```python
from build123d import *

# Parameters (mm, degrees)
PAD_DEPTH       = 3
SKETCH001_W     = 2
SKETCH001_H     = 6
POCKET_DEPTH    = 5
PAD001_DEPTH    = 2.2
SKETCH003_R     = 1.571244
POCKET001_DEPTH = 5


with BuildPart() as part:
    # Sketch → Pad (new body)
    with BuildSketch(Plane.XY):
        Polygon((0, -50), (9.32, -50), (9.32, 40), (35, 55), (35, 120), (0, 120), align=None)
    extrude(amount=PAD_DEPTH)

    # Sketch001 (on Face7 of Pad) → Pocket (cut)
    with BuildSketch(Plane(origin=(0, 0, 0), x_dir=(1, 0, 0), z_dir=(0, 0, -1))):
        with Locations((1, 0)):
            Rectangle(SKETCH001_W, SKETCH001_H)
    pocket = extrude(amount=-POCKET_DEPTH, mode=Mode.SUBTRACT)

    # Sketch002 (on Face3 of Pocket) → Pad001 (join)
    with BuildSketch(Plane.YZ.offset(9.32)):
        Polygon((-3, 0), (-3, 40), (-12, 40), (-34, 0), align=None)
    pad001 = extrude(amount=PAD001_DEPTH)

    # Sketch003 (on Face18 of Pad001) → Pocket001 (cut)
    with BuildSketch(Plane.YZ.offset(11.52)):
        with Locations((-8.751605, 34.485332)):
            Circle(SKETCH003_R)
    pocket001 = extrude(amount=-POCKET001_DEPTH, mode=Mode.SUBTRACT)

    # Mirrored: Pocket, Pad001, Pocket001 across XZ
    add(pocket.mirror(Plane.XZ), mode=Mode.SUBTRACT)
    add(pad001.mirror(Plane.XZ))
    add(pocket001.mirror(Plane.XZ), mode=Mode.SUBTRACT)


solid = part.part
```
Verification items for the finished model (mm, model axes). A direction names the side the tool comes from. Coordinates: 2 decimals unless noted, no trailing zeros. Order: outer loops, then holes, each group sorted by start corner. A loop starts at its lowest first (then second) coordinate and runs counter-clockwise, first axis right, second up. Notation, with made-up numbers: (63.25, 0) - (104.25, 0) arc R12 ccw to (104.25, 16) - close; hole circle Ø9 at (9.5, 51.5). An arc over 180 degrees is marked (long way). Return JSON: item names as keys, results as strings.
(1) Section check A-A, the plane z = 12. Record the cut outline in (x, y).
Filled sheet:
{"outline": "(9.32, -27.4) - (11.52, -27.4) - (11.52, -3) - (9.32, -3) - close; (9.32, 3) - (11.52, 3) - (11.52, 27.4) - (9.32, 27.4) - close"}
(2) Thickness scan on line 1 along Z through (x, y) = (27, 75); line 2 along Y through (x, z) = (11, 24.5) (3 decimals). Record the ranges inside material, lowest first.
Filled sheet:
{"line 1": "z = 0 to 3", "line 2": "y = -20.525 to -3, 3 to 20.525"}
(3) Section check B-B, the plane z = 28. Record the cut outline in (x, y).
Filled sheet:
{"outline": "(9.32, -18.6) - (11.52, -18.6) - (11.52, -3) - (9.32, -3) - close; (9.32, 3) - (11.52, 3) - (11.52, 18.6) - (9.32, 18.6) - close"}
(4) Go/stop test with flat-tipped pins: pin 1 (1.5 mm diameter, centred on y = -1, z = 2, fed in from -X); pin 2 (9 mm diameter, centred on y = -17.5, z = 30, fed in from -X); pin 3 (6 mm diameter, centred on x = 8, z = 8.5, fed in from -Y); pin 4 (2 mm diameter, centred on x = 7, z = 15.5, fed in from -Y). Record where each tip stops, or that it passes through.
Filled sheet:
{"pin 1": "stops at x = 2", "pin 2": "stops at x = 9.32", "pin 3": "stops at y = -30.81", "pin 4": "passes through"}
(5) Mould release check, pull along Y, two halves, no side actions. Record for faces 6 (the flat face through (10, -23, 20)), 7 (the flat face through (9.32, 36, 1)), 8 (the flat face through (18, 120, 1)), 9 (the flat face through (11.52, -15, 16)): pulls with the +Y half, pulls with the -Y half, needs draft (parallel to the pull), parting line crosses it, or undercut.
Filled sheet:
{"face 6": "pulls with the -Y half", "face 7": "undercut", "face 8": "pulls with the +Y half", "face 9": "needs draft"}
(6) Section check D-D, the plane x = 17. Record the cut outline in (y, z).
Filled sheet:
{"outline": "(44.49, 0) - (120, 0) - (120, 3) - (44.49, 3) - close"}
(7) Section check C-C, the plane y = 101.5. Record the cut outline in (x, z), and give its area (3 significant figures).
Filled sheet:
{"outline": "(0, 0) - (35, 0) - (35, 3) - (0, 3) - close", "area": "105 mm^2"}
(8) Access from +Z, -Z, +X, -X, +Y, -Y to the whole of each face (thin tool, end or side, straight path). Record for faces 1 (the flat face through (0, 62, 1)), 2 (the cylindrical face through (10.44, 9.09, 32.95)), 3 (the flat face through (9.32, -15, 18)), 4 (the flat face through (2, 0, 1)), 5 (the flat face through (9.32, 0, 1)).
Filled sheet:
{"face 1": "+Z, -Z, -X, +Y, -Y", "face 2": "+X, -X", "face 3": "+Z, -X, +Y, -Y", "face 4": "+Z, -Z, -X", "face 5": "+Z, -Z, +X"}
